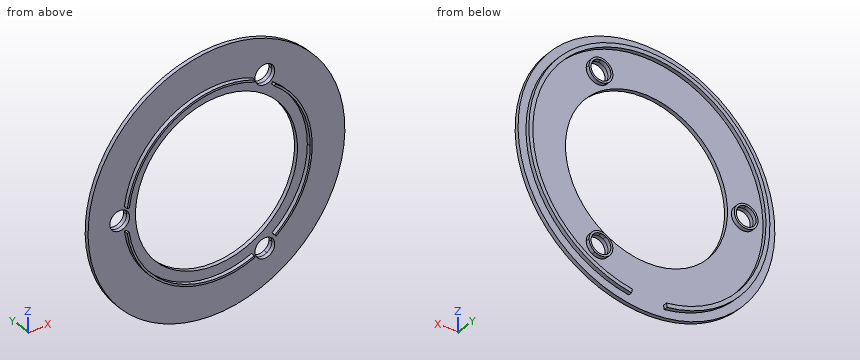
from build123d import *
from build123d.topology import SkipClean

# Parameters (mm, degrees)
CROQUIS1_R                 = 32.5
CROQUIS1_R_2               = 20.5
SALIENTE_EXTRUIR1_DEPTH    = 2
CORTAR_EXTRUIR1_START      = -1
CROQUIS2_R                 = 4.5
CROQUIS2_R_2               = 32.5
CROQUIS2_R_3               = 30.5
CROQUIS2_R_4               = 29.5
CORTAR_EXTRUIR1_DEPTH      = 1
SALIENTE_EXTRUIR2_DEPTH    = 1
CORTAR_EXTRUIR2_DEPTH      = 29
CORTAR_EXTRUIR2_DEPTH_BACK = 25
CROQUIS6_R                 = 2.5
SALIENTE_EXTRUIR3_DEPTH    = 1


with BuildPart() as part:
    # Croquis1 → Saliente-Extruir1 (new body)
    with BuildSketch(Plane(origin=(0, 0, 0), x_dir=(1, 0, 0), z_dir=(0, 1, 0))):
        with Locations(Location((0, 0, 0), (0, 0, 270))):
            Circle(CROQUIS1_R)
        with Locations(Location((0, 0, 0), (0, 0, 270))):
            Circle(CROQUIS1_R_2, mode=Mode.SUBTRACT)
    extrude(amount=SALIENTE_EXTRUIR1_DEPTH)

    # Croquis2 → Cortar-Extruir1 (cut)
    # profile 1 of 3: a face of its own
    with BuildSketch(Plane(origin=(0, 2, 0), x_dir=(1, 0, 0), z_dir=(0, 1, 0)).offset(CORTAR_EXTRUIR1_START)):
        with Locations((0, 30.5)):
            Circle(CROQUIS2_R)
    # profile 2 of 3: a face of its own
    with BuildSketch(Plane(origin=(0, 2, 0), x_dir=(1, 0, 0), z_dir=(0, 1, 0)).offset(CORTAR_EXTRUIR1_START)):
        with Locations(Location((0, 0, 0), (0, 0, 270))):
            Circle(CROQUIS2_R_2)
        Circle(CROQUIS2_R_3, mode=Mode.SUBTRACT)
    # profile 3 of 3: a face of its own
    with BuildSketch(Plane(origin=(0, 2, 0), x_dir=(1, 0, 0), z_dir=(0, 1, 0)).offset(CORTAR_EXTRUIR1_START)):
        Circle(CROQUIS2_R_4)
    extrude(amount=CORTAR_EXTRUIR1_DEPTH, mode=Mode.SUBTRACT)

    # Croquis3 → Saliente-Extruir2 (add)
    with BuildSketch(Plane(origin=(0, 1, 0), x_dir=(1, 0, 0), z_dir=(0, 1, 0))):
        with BuildLine():
            ThreePointArc((13.75, 23.815698604), (9.651923789, 22.717622393), (10.75, 18.619546181))
            Line((10.75, 18.619546181), (11, 19.052558883))
            ThreePointArc((11, 19.052558883), (10.084936491, 22.467622393), (13.5, 23.382685902))
            Line((13.5, 23.382685902), (13.75, 23.815698604))
        make_face()
        with BuildLine():
            Line((11, 19.052558883), (10.75, 18.619546181))
            ThreePointArc((10.75, 18.619546181), (13.75, 18.619546181), (15.25, 21.217622393))
            ThreePointArc((15.25, 21.217622393), (14.848076211, 22.717622393), (13.75, 23.815698604))
            Line((13.75, 23.815698604), (13.5, 23.382685902))
            ThreePointArc((13.5, 23.382685902), (14.415063509, 22.467622393), (14.75, 21.217622393))
            ThreePointArc((14.75, 21.217622393), (13.5, 19.052558883), (11, 19.052558883))
        make_face()
        with BuildLine():
            ThreePointArc((15.25, -21.217622393), (13.75, -18.619546181), (10.75, -18.619546181))
            Line((10.75, -18.619546181), (11, -19.052558883))
            ThreePointArc((11, -19.052558883), (13.5, -19.052558883), (14.75, -21.217622393))
            ThreePointArc((14.75, -21.217622393), (14.415063509, -22.467622393), (13.5, -23.382685902))
            Line((13.5, -23.382685902), (13.75, -23.815698604))
            ThreePointArc((13.75, -23.815698604), (14.848076211, -22.717622393), (15.25, -21.217622393))
        make_face()
        with BuildLine():
            Line((11, -19.052558883), (10.75, -18.619546181))
            ThreePointArc((10.75, -18.619546181), (9.651923789, -22.717622393), (13.75, -23.815698604))
            Line((13.75, -23.815698604), (13.5, -23.382685902))
            ThreePointArc((13.5, -23.382685902), (10.084936491, -22.467622393), (11, -19.052558883))
        make_face()
        with BuildLine():
            ThreePointArc((-27, 0), (-24.5, 2.5), (-22, 0))
            Line((-22, 0), (-21.5, 0))
            ThreePointArc((-21.5, 0), (-24.5, 3), (-27.5, 0))
            Line((-27.5, 0), (-27, 0))
        make_face()
        with BuildLine():
            Line((-21.5, 0), (-22, 0))
            ThreePointArc((-22, 0), (-24.5, -2.5), (-27, 0))
            Line((-27, 0), (-27.5, 0))
            ThreePointArc((-27.5, 0), (-24.5, -3), (-21.5, 0))
        make_face()
    extrude(amount=SALIENTE_EXTRUIR2_DEPTH)

    # Croquis6 → Cortar-Extruir2 (cut, two sides: drawn at the far end of the back side and taken through both)
    with SkipClean():  # the faces are left unmerged after this step: merging them gives an invalid solid
        with BuildSketch(Plane(origin=(0, 1, 0), x_dir=(1, 0, 0), z_dir=(0, 1, 0)).offset(-CORTAR_EXTRUIR2_DEPTH_BACK)):
            with Locations(Location((-24.5, 0, 0), (0, 0, 270))):
                Circle(CROQUIS6_R)
            with Locations(Location((12.25, -21.217622393, 0), (0, 0, 270))):
                Circle(CROQUIS6_R)
            with Locations(Location((12.25, 21.217622393, 0), (0, 0, 270))):
                Circle(CROQUIS6_R)
        extrude(amount=CORTAR_EXTRUIR2_DEPTH + CORTAR_EXTRUIR2_DEPTH_BACK, mode=Mode.SUBTRACT)

    # Croquis7 → Saliente-Extruir3 (add)
    with SkipClean():  # the faces are left unmerged after this step: merging them gives an invalid solid
        with BuildSketch(Plane.XZ):
            with BuildLine():
                ThreePointArc((9.061477105, 21.682703537), (-11.747329093, 20.353138804), (-23.307724042, 3))
                Line((-23.307724042, 3), (-22.803508502, 3))
                ThreePointArc((-22.803508502, 3), (-11.469500389, 19.936162139), (8.86867972, 21.221369419))
                Line((8.86867972, 21.221369419), (9.061477105, 21.682703537))
            make_face()
            with BuildLine():
                ThreePointArc((23.5, 0), (21.060096012, 10.427001294), (14.247033533, 18.688821137))
                Line((14.247033533, 18.688821137), (13.94390516, 18.291186645))
                ThreePointArc((13.94390516, 18.291186645), (20.612008862, 10.205150203), (23, 0))
                ThreePointArc((23, 0), (20.643150988, -10.142007557), (14.055624583, -18.20547768))
                Line((14.055624583, -18.20547768), (14.36118164, -18.601248934))
                ThreePointArc((14.36118164, -18.601248934), (21.09191514, -10.362485982), (23.5, 0))
            make_face()
            with BuildLine():
                Line((-22.803508502, -3), (-23.307724042, -3))
                ThreePointArc((-23.307724042, -3), (-11.747329093, -20.353138804), (9.061477105, -21.682703537))
                Line((9.061477105, -21.682703537), (8.86867972, -21.221369419))
                ThreePointArc((8.86867972, -21.221369419), (-11.469500389, -19.936162139), (-22.803508502, -3))
            make_face()
        extrude(amount=SALIENTE_EXTRUIR3_DEPTH)


solid = part.part
Work out the finished part from the listing and answer in its coordinate system (mm). Coordinates: 2 decimals unless noted, no trailing zeros. Write each loop counter-clockwise with the first axis right and the second up, starting at its lowest first coordinate (ties: lowest second). Pieces come first, ordered by that corner, then holes. Notation, with made-up numbers: M 49,71.25 L 67,71.25 A16 ccw 67,96.25 Z; hole C 82.5,78 d5. An arc over 180 degrees is marked long. Use one line per item in the form item = value. Start each with the question number.
1. The part is cut by section A-A (x = 0). Give the vertices of the cut face in (y, z).
2. Each of these flat-tipped pins is pushed along its axis until it touches: P1, Ø3, axis at x = -24.5, z = 0, coming from the +Y side; P2, Ø2, axis at x = -8.5, z = 23, coming from the +Y side; P3, Ø4, axis at x = 22.5, z = -16.5, coming from the -Y side. Where does it stop, or does it pass through?
3. The part is cut by section B-B (z = 6.5). Give the vertices of the cut face in (x, y).
4. The part is cut by section D-D (z = -27). Give the vertices of the cut face in (x, y).
5. Straight lines are drawn through the part: probe 1 along X at (y, z) = (0.3, 0); probe 2 along Z at (x, y) = (-24.5, 1.7); probe 3 along Z at (x, y) = (0, 1.6). For each, find the intervals that lie inside material, in ascending order. Write a range as from..to.
6. The part is cut by section C-C (x = -13.5). Give the vertices of the cut face in (y, z), plus the area to 3 significant figures.
Evaluation:
q1.outline = M -1,-23.5 L 0,-23.5 L 0,-32.5 L 1,-32.5 L 1,-20.5 L 0,-20.5 L 0,-23 L -1,-23 Z; M -1,23 L 0,23 L 0,20.5 L 1,20.5 L 1,29.5 L 2,29.5 L 2,30.5 L 1,30.5 L 1,32.5 L 0,32.5 L 0,23.5 L -1,23.5 Z
q2.P1 = through
q2.P2 = 1
q2.P3 = 0
q3.outline = M -31.84,0 L -22.58,0 L -22.58,-1 L -22.06,-1 L -22.06,0 L -19.44,0 L -19.44,1 L -28.77,1 L -28.77,2 L -29.8,2 L -29.8,1 L -31.84,1 Z; M 19.44,0 L 22.06,0 L 22.06,-1 L 22.58,-1 L 22.58,0 L 31.84,0 L 31.84,1 L 29.8,1 L 29.8,2 L 28.77,2 L 28.77,1 L 19.44,1 Z
q4.outline = M -18.09,0 L 18.09,0 L 18.09,1 L 14.19,1 L 14.19,2 L 11.88,2 L 11.88,1 L -11.88,1 L -11.88,2 L -14.19,2 L -14.19,1 L -18.09,1 Z
q5.probe_1 = -32.5..-27, -22..-20.5, 20.5..32.5
q5.probe_2 = -18.17..-16.43, -3..-2.5, 2.5..3, 16.43..18.17
q5.probe_3 = 29.5..30.5
q6.outline = M -1,-19.24 L 0,-19.24 L 0,-29.56 L 1,-29.56 L 1,-27.35 L 2,-27.35 L 2,-26.23 L 1,-26.23 L 1,-15.43 L 0,-15.43 L 0,-18.62 L -1,-18.62 Z; M -1,18.62 L 0,18.62 L 0,15.43 L 1,15.43 L 1,26.23 L 2,26.23 L 2,27.35 L 1,27.35 L 1,29.56 L 0,29.56 L 0,19.24 L -1,19.24 Z
q6.area = 31.7 mm^2
